from build123d import *

# Parameters (mm, degrees)
F1_DEPTH  = 63.5
F2_DEPTH  = 25.4
F3_DEPTH  = 8.255
F3_FACE_W = 17.145
F3_FACE_H = 19.05
F5_R      = 5.08


with BuildPart() as f1:
    # F0 (on Front) → F1 (new body, symmetric)
    with BuildSketch(Plane.XZ):
        Polygon((22.225, 9.525), (-41.275, 9.525), (-41.275, -9.525), (41.275, -9.525), (41.275, 9.525), align=None)
    extrude(amount=F1_DEPTH, both=True)

    # F0 (on Front) → F2 (join, symmetric)
    with BuildSketch(Plane.XZ):
        with BuildLine():
            Line((22.225, 27.0002), (22.225, 9.525))
            Line((22.225, 9.525), (41.275, 9.525))
            Line((41.275, 9.525), (41.275, 27.0002))
            ThreePointArc((41.275, 27.0002), (45.9246798487, 38.2255201513), (57.15, 42.8752))
            Line((57.15, 42.8752), (88.5989319826, 42.8752))
            Line((88.5989319826, 42.8752), (88.5989319826, 61.9252))
            Line((88.5989319826, 61.9252), (78.620570292, 61.9252))
            add(Edge.make_bspline(
                [(78.620570292, 61.9252), (68.1221807027, 61.8456885377), (58.0598709285, 61.5059481055), (48.5414196568, 60.8476219029)],
                knots=[6.3360896089, 6.3360896089, 6.3360896089, 6.3360896089, 26.5881828435, 26.5881828435, 26.5881828435, 26.5881828435], degree=3))
            ThreePointArc((48.5414196568, 60.8476219029), (29.5781820196, 48.4373284984), (22.225, 27.0002))
        make_face()
    extrude(amount=F2_DEPTH, both=True)

    # F0 (on Front) → F3 (join, symmetric)
    with BuildSketch(Plane.XZ):
        with BuildLine():
            add(Edge.make_bspline(
                [(48.5414196568, 60.8476219029), (-4.783802037, 57.1594808708), (-41.0396070564, 43.4722808258), (-41.275, 9.525)],
                knots=[26.5881828435, 26.5881828435, 26.5881828435, 26.5881828435, 140.0464893122, 140.0464893122, 140.0464893122, 140.0464893122], degree=3))
            Line((-41.275, 9.525), (22.225, 9.525))
            Line((22.225, 9.525), (22.225, 27.0002))
            ThreePointArc((22.225, 27.0002), (29.5781820196, 48.4373284984), (48.5414196568, 60.8476219029))
        make_face()
        Polygon((22.225, 9.525), (-41.275, 9.525), (-41.275, -9.525), (41.275, -9.525), (41.275, 9.525), align=None)
        with BuildLine():
            Line((22.225, 27.0002), (22.225, 9.525))
            Line((22.225, 9.525), (41.275, 9.525))
            Line((41.275, 9.525), (41.275, 27.0002))
            ThreePointArc((41.275, 27.0002), (45.9246798487, 38.2255201513), (57.15, 42.8752))
            Line((57.15, 42.8752), (88.5989319826, 42.8752))
            Line((88.5989319826, 42.8752), (88.5989319826, 61.9252))
            Line((88.5989319826, 61.9252), (78.620570292, 61.9252))
            add(Edge.make_bspline(
                [(78.620570292, 61.9252), (68.1221807027, 61.8456885377), (58.0598709285, 61.5059481055), (48.5414196568, 60.8476219029)],
                knots=[6.3360896089, 6.3360896089, 6.3360896089, 6.3360896089, 26.5881828435, 26.5881828435, 26.5881828435, 26.5881828435], degree=3))
            ThreePointArc((48.5414196568, 60.8476219029), (29.5781820196, 48.4373284984), (22.225, 27.0002))
        make_face()
        with BuildLine():
            ThreePointArc((57.15, 61.9252), (52.8121194668, 61.6547583939), (48.5414196568, 60.8476219029))
            add(Edge.make_bspline(
                [(78.620570292, 61.9252), (68.1221807027, 61.8456885377), (58.0598709285, 61.5059481055), (48.5414196568, 60.8476219029)],
                knots=[6.3360896089, 6.3360896089, 6.3360896089, 6.3360896089, 26.5881828435, 26.5881828435, 26.5881828435, 26.5881828435], degree=3))
            Line((78.620570292, 61.9252), (57.15, 61.9252))
        make_face()
        with BuildLine():
            add(Edge.make_bspline(
                [(88.5989319826, 61.9252), (85.23232743, 61.9494803379), (81.9051066812, 61.9500760335), (78.620570292, 61.9252)],
                knots=[0, 0, 0, 0, 6.3360896089, 6.3360896089, 6.3360896089, 6.3360896089], degree=3))
            Line((78.620570292, 61.9252), (88.5989319826, 61.9252))
        make_face()
        Polygon((88.5989319826, 66.675), (88.5989319826, 61.9252), (88.5989319826, 42.8752), (88.5989319826, 38.1), (139.3989319826, 38.1), (139.3989319826, 66.675), align=None)
    extrude(amount=F3_DEPTH, both=True)

    # F3_face (on face) → F4 (revolve)
    with BuildSketch(Plane(origin=(88.5989319826, 16.8275, 52.4002), x_dir=(0, 1, 0), z_dir=(1, 0, 0))):
        Rectangle(F3_FACE_W, F3_FACE_H)
    revolve(axis=Axis((88.5989319826, -8.255, 52.4002), (0, 0, 1)))

    # F5
    f5_edges = [f1.edges().sort_by_distance(p)[0] for p in [
        (-41.275, -63.5, 0),
        (41.275, -63.5, 0),
        (41.275, 63.5, 0),
        (-41.275, 63.5, 0),
    ]]
    fillet(f5_edges, radius=F5_R)


solid = f1.part
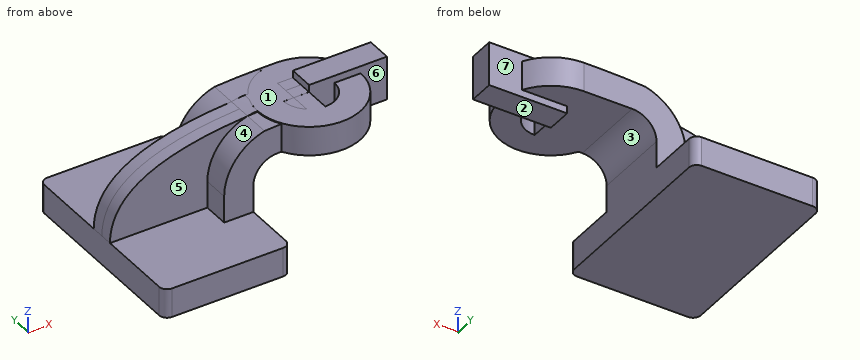
Work out the finished part from the listing and answer in its coordinate system (mm). Face numbers are marked on the shaded views. A direction names the side the tool comes from. Round coordinates to 2 decimals unless told otherwise and drop trailing zeros. Order: outer loops, then holes, each group sorted by start corner. A loop starts at its lowest first (then second) coordinate and runs counter-clockwise, first axis right, second up. Notation, with made-up numbers: M -21,-27.5 L 18,-27.5 A27 cw 18,7.5 Z; hole C 4.5,-20 d3. An arc over 180 degrees is marked long. Put each result on its own line as item: value. Start each with the question number.
Q1. Section D-D, the plane x = 115.5 is taken. Write down the section's boundary in (y, z) (3 decimals).
Q2. Straight lines are drawn through the part: L1, parallel to Y at x = 20, z = 14.5 (3 decimals); L2, parallel to Z at x = 16, y = -21.5 (3 decimals); L3, parallel to Z at x = 79.5, y = -34.5. For each, find the intervals that lie inside material, in ascending order. Write a range as [from, to].
Q3. Section B-B, the plane y = -37 is taken. Write down the section's boundary in (x, z) (3 decimals).
Q4. Flat-ended cylindrical pins translate along their axes: pin 1 (5 mm diameter, centred on y = -19.5, z = 19, fed in from -X) (3 decimals); pin 2 (0.5 mm diameter, centred on x = 52, z = 61.5, fed in from -Y) (3 decimals); pin 3 (23 mm diameter, centred on x = 110, z = 59, fed in from +Y); pin 4 (18 mm diameter, centred on y = -15.5, z = 55, fed in from +X). Find the tip coordinate at first contact, or state that the pin passes through.
Q5. For a pull along Y with two mould halves and no side action, classify the marked faces 5, 6 and 7 as pulls with the +Y half, pulls with the -Y half, needs draft (parallel to the pull), parting line crosses it, or undercut.
Q6. Section A-A, the plane x = 95 is taken. Write down the section's boundary in (y, z) (3 decimals), and give its area (3 significant figures).
Q7. Section C-C, the plane z = -1.5 is taken. Write down the section's boundary in (x, y) (3 decimals), and give its area (3 significant figures).
Q8. A tool of negligible diameter and unlimited length cuts with its end or side. For the marked faces 1, 2, 3 and 4, from which of +Z, -Z, +X, -X, +Y, -Y can it reach the whole face along a straight path? Write none if from no direction.
Findings below:
1. outline: M -28.479,42.875 L -8.255,42.875 L -8.255,38.1 L 8.255,38.1 L 8.255,42.875 L 11.969,42.875 L 11.969,61.925 L 8.255,61.925 L 8.255,66.675 L -8.255,66.675 L -8.255,61.925 L -28.479,61.925 Z
2. L1: y = [-8.255, 8.255]
2. L2: z = [-9.525, 9.525]
2. L3: z = [42.88, 61.93]
3. outline: M -41.275,-9.525 L 41.275,-9.525 L 41.275,9.525 L -41.275,9.525 Z; M 71.095,42.875 L 106.103,42.875 L 106.103,61.925 L 71.095,61.925 Z
4. pin 1: stops at x = 22.225
4. pin 2: stops at y = -8.255
4. pin 3: stops at y = 23.91
4. pin 4: stops at x = 139.4
5. face 5: pulls with the -Y half
5. face 6: undercut
5. face 7: pulls with the +Y half
6. outline: M -41.296,42.875 L -23.474,42.875 L -23.474,61.925 L -41.296,61.925 Z; M -8.255,38.1 L 8.255,38.1 L 8.255,42.875 L 24.786,42.875 L 24.786,61.925 L 8.255,61.925 L 8.255,66.675 L -8.255,66.675 Z
6. area: 1,130 mm^2
7. outline: M -41.275,-58.42 A5.08 ccw -36.195,-63.5 L 36.195,-63.5 A5.08 ccw 41.275,-58.42 L 41.275,58.42 A5.08 ccw 36.195,63.5 L -36.195,63.5 A5.08 ccw -41.275,58.42 Z
7. area: 10,500 mm^2
8. face 1: +Z, -X
8. face 2: -Z, +X, +Y, -Y
8. face 3: -Z, +Y, -Y
8. face 4: +Z, -X, -Y
